Work out the finished part from the listing and answer in its coordinate system (mm). Face numbers are marked on the shaded views. Round coordinates to 2 decimals unless told otherwise and drop trailing zeros. Order: outer loops, then holes, each group sorted by start corner. A loop starts at its lowest first (then second) coordinate and runs counter-clockwise, first axis right, second up. Notation, with made-up numbers: M 83,2 L 103,2 A21 ccw 103,24 Z; hole C -27.75,-37 d11. An arc over 180 degrees is marked long. Answer as a JSON object with one key per item and string values. Group by question number.
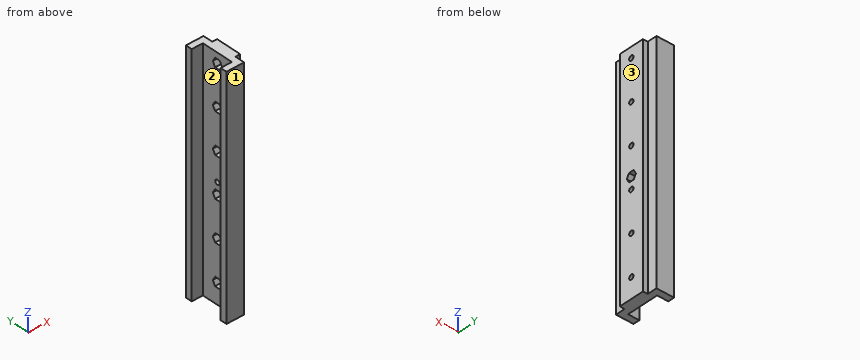
from build123d import *

# Parameters (mm, degrees)
PAD034_DEPTH            = 144
SKETCH063_R             = 1.5
POCKET027_DEPTH         = 7
POCKET028_DEPTH         = 4
SKETCH067_R             = 1.5
POCKET031_DEPTH         = 7
POCKET032_DEPTH         = 5
BODY019_ROLL_ANGLE      = 90
BODY019_PLACEMENT_ANGLE = 180


with BuildPart() as rightlow:
    # Sketch062 → Pad034 (new body)
    with BuildSketch(Plane.XZ):
        Polygon((0, 0), (0, 10), (-7, 10), (-7, 14), (4, 14), (4, 8), (7, 8), (7, -8), (4, -8), (4, -14), (-7, -14), (-7, -10), (0, -10), align=None)
    extrude(amount=PAD034_DEPTH)

    # Sketch063 (on Face6 of Pad034) → Pocket027 (cut)
    with BuildSketch(Plane(origin=(7, 0, 0), x_dir=(0, 0, 1), z_dir=(1, 0, 0))):
        with Locations((0, 74)):
            Circle(SKETCH063_R)
    extrude(amount=-POCKET027_DEPTH, mode=Mode.SUBTRACT)

    # Sketch064 (on Face11 of Pocket027) → Pocket028 (cut)
    with BuildSketch(Plane(origin=(7, 0, 0), x_dir=(0, 0, 1), z_dir=(1, 0, 0))):
        Polygon((3.176, 74.000007), (1.587994, 76.7505), (-1.588006, 76.750493), (-3.176, 73.999993), (-1.587994, 71.2495), (1.588006, 71.249507), align=None)
    extrude(amount=-POCKET028_DEPTH, mode=Mode.SUBTRACT)

    # Sketch067 (on Face2 of Pocket028) → Pocket031 (cut)
    with BuildSketch(Plane(origin=(0, 0, 0), x_dir=(0, 0, -1), z_dir=(-1, 0, 0))):
        with Locations((0, 131.5)):
            Circle(SKETCH067_R)
        with Locations((0, 106.5)):
            Circle(SKETCH067_R)
        with Locations((0, 56.5)):
            Circle(SKETCH067_R)
        with Locations((0, 31.5)):
            Circle(SKETCH067_R)
        with Locations((0, 6.5)):
            Circle(SKETCH067_R)
        with Locations((0, 81.5)):
            Circle(SKETCH067_R)
    extrude(amount=-POCKET031_DEPTH, mode=Mode.SUBTRACT)

    # Sketch068 → Pocket032 (cut)
    with BuildSketch(Plane(origin=(0, 0, 0), x_dir=(0, 0, -1), z_dir=(-1, 0, 0))):
        Polygon((3.175246, 131.569182), (1.52771, 134.284435), (-1.647536, 134.215253), (-3.175246, 131.430818), (-1.52771, 128.715565), (1.647536, 128.784747), align=None)
        Polygon((3.176, 106.5), (1.588, 109.250497), (-1.588, 109.250497), (-3.176, 106.5), (-1.588, 103.749503), (1.588, 103.749503), align=None)
        Polygon((3.176, 56.50001), (1.587991, 59.250502), (-1.588009, 59.250491), (-3.176, 56.49999), (-1.587991, 53.749498), (1.588009, 53.749509), align=None)
        Polygon((3.176, 31.499996), (1.588004, 34.250495), (-1.587996, 34.250499), (-3.176, 31.500004), (-1.588004, 28.749505), (1.587996, 28.749501), align=None)
        Polygon((3.176, 81.5), (1.588, 84.250497), (-1.588, 84.250497), (-3.176, 81.5), (-1.588, 78.749503), (1.588, 78.749503), align=None)
        Polygon((3.176, 6.5), (1.588, 9.250497), (-1.588, 9.250497), (-3.176, 6.5), (-1.588, 3.749503), (1.588, 3.749503), align=None)
    extrude(amount=-POCKET032_DEPTH, mode=Mode.SUBTRACT)


with BuildPart() as rightlow_1:
    # Body019 roll: moved
    add(rightlow.part.rotate(Axis((0, 0, 0), (1, 0, 0)), BODY019_ROLL_ANGLE))


with BuildPart() as rightlow_2:
    # Body019 placement: moved
    add(rightlow_1.part.moved(Location((120, -275.5, 144))).rotate(Axis((120, -275.5, 144), (0, 0, 1)), BODY019_PLACEMENT_ANGLE))


with BuildPart() as leftlow:
    # Part__Mirroring008: instance of RightLow
    add(rightlow_2.part.mirror(Plane(origin=(0, 0, 0), x_dir=(0, -1, 0), z_dir=(1, 0, 0))))


solid = leftlow.part
Item 1: The mould has two halves that part along Y. Classify the marked faces 1, 2 and 3: +Y half, -Y half, draft (parallel to the pull), parting line (faces both ways), or undercut.
Item 2: Find section C-C (y = -275.5). Give the number of separate pieces and of enclosed holes in the cut face, and give its area (3 significant figures).
Item 3: Consider L1, parallel to Y at x = -113.6, z = 137.5; L2, parallel to Y at x = -122.75, z = 113.5; L3, parallel to X at y = -271, z = 31.5. Determine where each line is inside the solid, lowest interval first.
Item 4: Each of these flat-tipped pins is pushed along its axis until it touches: pin 1 (1.7 mm diameter, centred on y = -276.5, z = 71, fed in from +X); pin 2 (4.5 mm diameter, centred on y = -277, z = 62, fed in from -X); pin 3 (0.9 mm diameter, centred on x = -114, z = 73.5, fed in from -Y). Where does it stop, or does it pass through?
Item 5: Find section B-B (z = 33). Give the vertices of the cut face in (x, y), and give its area (3 significant figures).
Item 6: Find section A-A (x = -124.5). Give the vertices of the cut face in (y, z), and give its area (3 significant figures).
Responses:
{
 "1": {"face 1": "-Y half", "face 2": "undercut", "face 3": "draft"},
 "2": {"separate pieces": "8", "enclosed holes": "0", "area": "776 mm^2"},
 "3": {"L1": "y = -283.5 to -277, -274 to -267.5", "L2": "y = -289.5 to -285.5, -265.5 to -261.5", "L3": "x = -120 to -113"},
 "4": {"pin 1": "stops at x = -117", "pin 2": "stops at x = -120", "pin 3": "stops at y = -283.5"},
 "5": {"outline": "M -127,-289.5 L -116,-289.5 L -116,-283.5 L -113,-283.5 L -113,-267.5 L -116,-267.5 L -116,-261.5 L -127,-261.5 L -127,-265.5 L -120,-265.5 L -120,-285.5 L -127,-285.5 Z", "area": "216 mm^2"},
 "6": {"outline": "M -289.5,0 L -285.5,0 L -285.5,144 L -289.5,144 Z; M -265.5,0 L -261.5,0 L -261.5,144 L -265.5,144 Z", "area": "1,150 mm^2"}
}
